Autodesk Inventor part; units mm, degrees
ref_plane "YZ Plane" through (0, 0, 0) normal (1, 0, 0) x (0, 1, 0)
ref_plane "XZ Plane" through (0, 0, 0) normal (0, 1, 0) x (-1, 0, 0)
ref_plane "XY Plane" through (0, 0, 0) normal (0, 0, 1) x (1, 0, 0)
sketch "Skizze3" plane through (0, 0, 0) normal (1, 0, 0) x (0, 1, 0)
  line L0 (0, 0) -> (6.2939, 0)
  line L1 (0, 6) -> (0, 4)
  line L2 (0, 4) -> (1, 4)
  line L3 (1, 4) -> (1, 2.5)
  line L4 (1, 2.5) -> (3, 2.5)
  line L5 (3, 2.5) -> (3, 6)
  line L6 (3, 6) -> (0, 6)
  dimension "d4" = 12
  dimension "d5" = 5
  dimension "d6" = 3
  dimension "d7" = 1
  dimension "d9" = 8
revolve "Umdrehung1" add sketch "Skizze3" angle 360 about axis through (0, 0, 0) along (0, 1, 0)
chamfer "Fase1" distance 0.2 angle 45 4 edges at (0, 3, -6) (0, 0, -6) (0, 3, -2.5) (0, 1, -2.5)
properties part number "BT013_huenin20_23" material "Gummi"
The model under review builds one solid part; all positions refer to its coordinate system, in mm. A direction names the side the tool comes from. Coordinates: 2 decimals unless noted, no trailing zeros. Order: outer loops, then holes, each group sorted by start corner. A loop starts at its lowest first (then second) coordinate and runs counter-clockwise, first axis right, second up. Notation, with made-up numbers: (-15, 21.5) -> (42, 21.5) arc R33 cw to (42, 51.5) -> close; hole circle Ø6 at (69, 75). An arc over 180 degrees is marked (long way). Answer in a Markdown table with one row per item. Add a question column.
Item 1: Mouldability with a two-part tool opening along X and no side actions: class faces 3 (the flat face through (3.95, 0, -1.37)), 4 (the cylindrical face through (0, 1, -6)), 5 (the cylindrical face through (-3.905, 0.507, -0.867)) as +X half, -X half, draft (parallel to the pull), parting line (faces both ways), or undercut.
Item 2: Clearance check with flat-ended pins moving along their axes: pin 1 (2.5 mm diameter, centred on x = 0, z = -2, fed in from -Y); pin 2 (1 mm diameter, centred on x = 3.5, y = 2.5, fed in from -Z). State where each tip first meets the part, or that it passes through.
Item 3: To check wall thickness, follow probe 1 along X at (y, z) = (0.55, 0); probe 2 along X at (y, z) = (2.4, 0); probe 3 along Z at (x, y) = (-2, 2.2). State the ranges of each line that lie inside material, in increasing order.
Item 4: We need section C-C on y = 1.4. Write out the cut boundary in (x, z).
Item 5: We need section B-B on z = 0. Write out the cut boundary in (x, y), plus the area to 3 significant figures.
Item 6: We need section D-D on y = 0.5. Write out the cut boundary in (x, z), plus the area to 3 significant figures.
Item 7: We need section A-A on x = 0. Write out the cut boundary in (y, z), plus the area to 3 significant figures.
Item 8: Machinability: for faces 1 (the flat face through (-1, 1, 3)), 2 (the flat face through (1.4, 3, 2.5)), which of the approach directions +Z, -Z, +X, -X, +Y, -Y give a long, thin tool a straight path to every point of the face, cutting with its end or side? Answer none if there is none.
Final values:
| question | item | result |
|---|---|---|
| 1 | face 3 | draft |
| 1 | face 4 | parting line |
| 1 | face 5 | undercut |
| 2 | pin 1 | stops at y = 1 |
| 2 | pin 2 | stops at z = -5.2 |
| 3 | probe 1 | x = -6 to -4, 4 to 6 |
| 3 | probe 2 | x = -6 to -2.5, 2.5 to 6 |
| 3 | probe 3 | z = -5.66 to -1.5, 1.5 to 5.66 |
| 4 | outline | circle Ø12 at (0, 0); hole circle Ø5 at (0, 0) |
| 5 | outline | (-6, 0.2) -> (-5.8, 0) -> (-4, 0) -> (-4, 1) -> (-2.7, 1) -> (-2.5, 1.2) -> (-2.5, 2.8) -> (-2.7, 3) -> (-5.8, 3) -> (-6, 2.8) -> close; (2.5, 1.2) -> (2.7, 1) -> (4, 1) -> (4, 0) -> (5.8, 0) -> (6, 0.2) -> (6, 2.8) -> (5.8, 3) -> (2.7, 3) -> (2.5, 2.8) -> close |
| 5 | area | 17.8 mm2 |
| 6 | outline | circle Ø12 at (0, 0); hole circle Ø8 at (0, 0) |
| 6 | area | 62.8 mm2 |
| 7 | outline | (0, -5.8) -> (0.2, -6) -> (2.8, -6) -> (3, -5.8) -> (3, -2.7) -> (2.8, -2.5) -> (1.2, -2.5) -> (1, -2.7) -> (1, -4) -> (0, -4) -> close; (0, 4) -> (1, 4) -> (1, 2.7) -> (1.2, 2.5) -> (2.8, 2.5) -> (3, 2.7) -> (3, 5.8) -> (2.8, 6) -> (0.2, 6) -> (0, 5.8) -> close |
| 7 | area | 17.8 mm2 |
| 8 | face 1 | -Y |
| 8 | face 2 | +Z, -Z, +X, -X, +Y |
